Read the model definition and answer for the solid it produces. Units are mm, in the model's axes. Face numbers are marked on the shaded views. A direction names the side the tool comes from. Give positions to 0.01 mm unless a question says otherwise; leave off trailing zeros. Order: outer loops, then holes, each group sorted by start corner. A loop starts at its lowest first (then second) coordinate and runs counter-clockwise, first axis right, second up. Notation, with made-up numbers: (84.5, 3.5) - (133.5, 3.5) arc R22 cw to (133.5, 14.5) - close; hole circle Ø2 at (36.25, 69). An arc over 180 degrees is marked (long way). Write item = value, one per line.
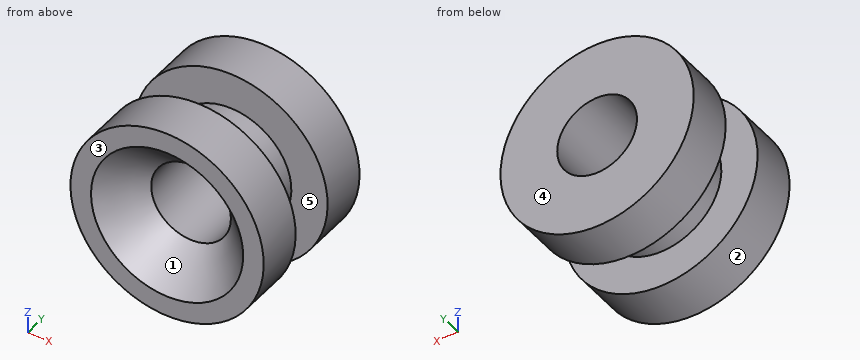
```python
from build123d import *

# Parameters (mm, degrees)
CSK_FOR_M6_FLAT_HEAD_MACHINE_SCREW1_D           = 6.6
CSK_FOR_M6_FLAT_HEAD_MACHINE_SCREW1_CSINK_D     = 12.6
CSK_FOR_M6_FLAT_HEAD_MACHINE_SCREW1_CSINK_ANGLE = 90


with BuildPart() as part:
    # Sketch1 → Revolve1 (revolve)
    with BuildSketch(Plane.XY, mode=Mode.PRIVATE) as revolve1_sk:
        Polygon((0, 0), (0, -6), (-8, -6), (-8, -2), (-5, -2), (-5, 0), align=None)
    revolve(revolve1_sk.sketch.rotate(Axis((0, 0, 0), (0, -1, 0)), 270), axis=Axis((0, 0, 0), (0, -1, 0)))

    # Mirror1: part across plane


with BuildPart() as part_1:
    add(part.part)
    add(part.part.mirror(Plane(origin=(-5, 0, 0), x_dir=(0, 0, 1), z_dir=(0, 1, 0))))

    # CSK for M6 Flat Head Machine Screw1 (through all)
    with Locations(Plane(origin=(0, -6, 0), x_dir=(-1, 0, 0), z_dir=(0, -1, 0))):
        with Locations((0, 0)):
            CounterSinkHole(CSK_FOR_M6_FLAT_HEAD_MACHINE_SCREW1_D / 2, CSK_FOR_M6_FLAT_HEAD_MACHINE_SCREW1_CSINK_D / 2, counter_sink_angle=CSK_FOR_M6_FLAT_HEAD_MACHINE_SCREW1_CSINK_ANGLE)


solid = part_1.part
```
1. Straight lines are drawn through the part: L1, parallel to Y at x = 7, z = 3; L2, parallel to X at y = 4, z = -2; L3, parallel to Y at x = -0.5, z = -6. For each, find the intervals that lie inside material, in ascending order. Write a range as [from, to].
Recorded:
L1 = [-6, -2], [2, 6]
L2 = [-7.75, -2.62], [2.62, 7.75]
L3 = [-5.72, -2], [2, 6]
2. Section B-B (x = 0) is taken. Determine the outline of the cut face in (y, z), and give its area (3 significant figures).
Recorded:
outline = (-6, -8) - (-2, -8) - (-2, -5) - (2, -5) - (2, -8) - (6, -8) - (6, -3.3) - (-3, -3.3) - (-6, -6.3) - close; (-6, 6.3) - (-3, 3.3) - (6, 3.3) - (6, 8) - (2, 8) - (2, 5) - (-2, 5) - (-2, 8) - (-6, 8) - close
area = 79.8 mm^2
3. Determine the mould class of the marked faces 1, 2 and 3 for opening direction Z: +Z half, -Z half, draft (parallel to the pull), parting line (faces both ways), or undercut.
Recorded:
face_1 = undercut
face_2 = parting line
face_3 = draft
4. Section D-D (y = -3.5) is taken. Determine the outline of the cut face in (x, z), and give its area (3 significant figures).
Recorded:
outline = circle Ø16 at (0, 0); hole circle Ø7.6 at (0, 0)
area = 156 mm^2
5. For the marked faces 4 and 5, determine the directions among +Z, -Z, +X, -X, +Y, -Y from which every point of the face is accessible in a straight line to the end or side of a thin tool.
Recorded:
face_4 = +Z, -Z, +X, -X, +Y
face_5 = none
6. Section A-A (z = 0) is taken. Determine the outline of the cut face in (x, y), and give its area (3 significant figures).
Recorded:
outline = (-8, -6) - (-6.3, -6) - (-3.3, -3) - (-3.3, 6) - (-8, 6) - (-8, 2) - (-5, 2) - (-5, -2) - (-8, -2) - close; (3.3, -3) - (6.3, -6) - (8, -6) - (8, -2) - (5, -2) - (5, 2) - (8, 2) - (8, 6) - (3.3, 6) - close
area = 79.8 mm^2
7. Flat-ended cylindrical pins translate along their axes: pin 1 (5 mm diameter, centred on x = -3, z = 1.5, fed in from -Y); pin 2 (2 mm diameter, centred on y = -1.5, z = -5, fed in from +X); pin 3 (1.5 mm diameter, centred on y = -3, z = 2, fed in from -X). Find the tip coordinate at first contact, or state that the pin passes through.
Recorded:
pin_1 = -5.55
pin_2 = 6.85
pin_3 = -7.9
8. Section C-C (y = 1.75) is taken. Determine the outline of the cut face in (x, z).
Recorded:
outline = circle Ø10 at (0, 0); hole circle Ø6.6 at (0, 0)
